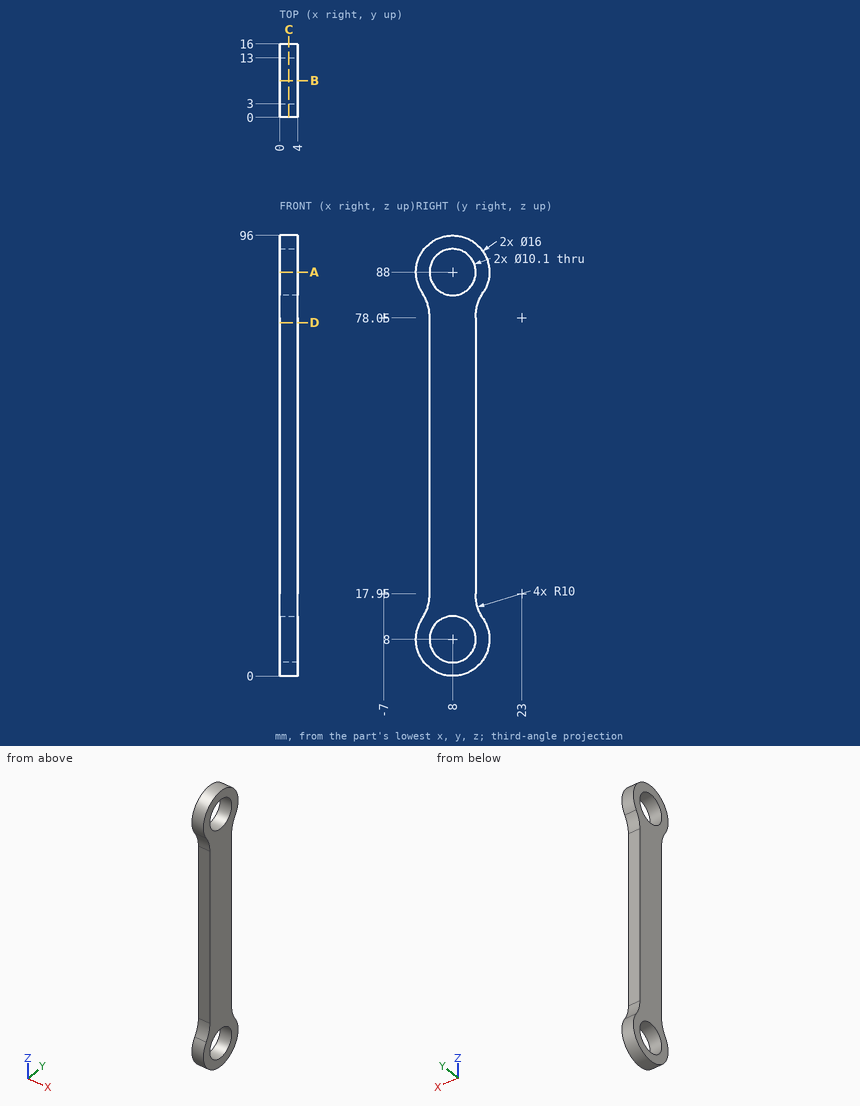
Input: dimensioned drawing with shaded views. Units: mm. Origin: part minimum x, y, z. Give positions to 0.01 mm unless a question says otherwise; leave off trailing zeros. Loops run counter-clockwise (first coordinate to the right, second up) from the corner with the lowest first, then second, coordinate; pieces in that order, holes last. Notation, with made-up numbers: (-25.5, -22.75) -> (-5.5, -22.75) arc R18 ccw to (-5.5, 1.25) -> close; hole circle Ø7 at (76.5, -16). An arc over 180 degrees is marked (long way). Use a Markdown table: item, result. Add a question column.
1) Section query B-B, the plane y = 8. Return the cut outline in (x, z).
2) Section query D-D, the plane z = 77. Return the cut outline in (x, y).
3) First-contact query: pin 1 (2 mm diameter, centred on x = 3, z = 36.5, fed in from -Y); pin 2 (2 mm diameter, centred on x = 1.5, y = 10.5, fed in from -Z); pin 3 (1.5 mm diameter, centred on x = 2, y = 14, fed in from +Z); pin 4 (1.5 mm diameter, centred on y = 2, z = 76, fed in from +X). Flat tips, straight axial feed; report the tip coordinate or a pass-through.
4) Section query A-A, the plane z = 88. Return the cut outline in (x, y).
5) Section query C-C, the plane x = 2. Return the cut outline in (y, z).
6) Line query: line 1 along Z through (x, y) = (2.05, 8); line 2 along Z through (x, y) = (0.9, 12); line 3 along Y through (x, z) = (3, 88). Output: solid intervals per line, ascending. Write a range as [from, to].
Numbers:
| question | item | result |
|---|---|---|
| 1 | outline | (0, 0) -> (4, 0) -> (4, 2.95) -> (0, 2.95) -> close; (0, 13.05) -> (4, 13.05) -> (4, 82.95) -> (0, 82.95) -> close; (0, 93.05) -> (4, 93.05) -> (4, 96) -> (0, 96) -> close |
| 2 | outline | (0, 3) -> (4, 3) -> (4, 13) -> (0, 13) -> close |
| 3 | pin 1 | stops at y = 3 |
| 3 | pin 2 | stops at z = 0.14 |
| 3 | pin 3 | stops at z = 94.04 |
| 3 | pin 4 | passes through |
| 4 | outline | (0, 0) -> (4, 0) -> (4, 2.95) -> (0, 2.95) -> close; (0, 13.05) -> (4, 13.05) -> (4, 16) -> (0, 16) -> close |
| 5 | outline | (1.33, 12.42) arc R8 ccw (long way) to (14.67, 12.42) arc R10 cw to (13, 17.95) -> (13, 78.05) arc R10 cw to (14.67, 83.58) arc R8 ccw (long way) to (1.33, 83.58) arc R10 cw to (3, 78.05) -> (3, 17.95) arc R10 cw to start; hole circle Ø10.1 at (8, 8); hole circle Ø10.1 at (8, 88) |
| 6 | line 1 | z = [0, 2.95], [13.05, 82.95], [93.05, 96] |
| 6 | line 2 | z = [1.07, 4.92], [11.08, 84.92], [91.08, 94.93] |
| 6 | line 3 | y = [0, 2.95], [13.05, 16] |
